The listing builds one solid part. Answer for the finished solid, in the listing's coordinates (mm). A direction names the side the tool comes from. Round coordinates to 2 decimals unless told otherwise and drop trailing zeros. Loops run counter-clockwise (first coordinate to the right, second up) from the corner with the lowest first, then second, coordinate; pieces in that order, holes last. Notation, with made-up numbers: (10.25, -23.5) -> (68.25, -23.5) arc R15 cw to (68.25, 0.5) -> close; hole circle Ø5 at (-6.5, -22). An arc over 180 degrees is marked (long way). Use a Markdown table: item, result. Add a question column.
Q1. Section C-C on y = -10 is taken. Give the vertices of the cut face in (x, z).
Q2. Given pin 1 Ø2 at (y, z) = (31.5, 4) entering from -X; pin 2 Ø3 at (y, z) = (14.5, -5.5) entering from -X; pin 3 Ø5 at (x, z) = (1.5, 4) entering from -Y, each flat-ended and moving along its own axis, determine where each tip first touches the part or whether it passes through.
Q3. Section D-D on z = -7 is taken. Give the vertices of the cut face in (x, y).
Q4. Section B-B on x = -2 is taken. Give the vertices of the cut face in (y, z).
Q5. Consider line 1 (Y direction, x = 0, z = -0.1); line 2 (Y direction, x = 4.5, z = -7); line 3 (Y direction, x = 2.25, z = 1). Determine where each line is inside the solid, lowest interval first.
Q6. Which of the six approach directions +Z, -Z, +X, -X, +Y, -Y give full straight-line access (tool end or side, diameter ignored) to faces 5 (the flat face through (0, -8, 0.75)), 6 (the flat face through (0, -12, 0)), 7 (the cylindrical face through (0.9, -0.99, -2.86))?
Q7. Section A-A on z = 0 is taken. Give the vertices of the cut face in (x, y).
Q8. For a pull along Y with two mould halves and no side action, classify faces 1 (the flat face through (0.1, 0, 3.4)), 2 (the flat face through (0, 39.5, 0)), 3 (the cylindrical face through (-0.108, -10.488, -0.31)), 4 (the cylindrical face through (-8.428, 28.092, 1.107)) as released by +Y, released by -Y, zero draft, split by the parting line, or undercut.
from build123d import *

# Parameters (mm, degrees)
SKETCH1_R               = 8
BOSS_EXTRUDE1_DEPTH     = 17
SKETCH2_R               = 8.5
BOSS_EXTRUDE2_DEPTH     = 22.5
SKETCH3_R               = 3
BOSS_EXTRUDE3_DEPTH     = 2
SKETCH4_R               = 1.4
BOSS_EXTRUDE4_DEPTH     = 10
CUT_EXTRUDE1_START      = -8.5
CUT_EXTRUDE1_DEPTH      = 8.5
CUT_EXTRUDE2_REACH      = 43.45
CUT_EXTRUDE2_END_RADIUS = 1.4
SKETCH6_R               = 0.5


with BuildPart() as part:
    # Sketch1 → Boss-Extrude1 (new body)
    with BuildSketch(Plane(origin=(0, 0, 0), x_dir=(1, 0, 0), z_dir=(0, 1, 0))):
        with Locations(Location((0, 0, 0), (0, 0, 270))):
            Circle(SKETCH1_R)
    extrude(amount=BOSS_EXTRUDE1_DEPTH)

    # Sketch2 → Boss-Extrude2 (add)
    with BuildSketch(Plane(origin=(0, 17, 0), x_dir=(1, 0, 0), z_dir=(0, 1, 0))):
        with Locations(Location((0, 0, 0), (0, 0, 90))):
            Circle(SKETCH2_R)
    extrude(amount=BOSS_EXTRUDE2_DEPTH)

    # Sketch3 → Boss-Extrude3 (add)
    with BuildSketch(Plane.XZ):
        with Locations(Location((0, 0, 0), (0, 0, 270))):
            Circle(SKETCH3_R)
    extrude(amount=BOSS_EXTRUDE3_DEPTH)

    # Sketch4 → Boss-Extrude4 (add)
    with BuildSketch(Plane.XZ.offset(2)):
        with Locations(Location((0, 0, 0), (0, 0, 270))):
            Circle(SKETCH4_R)
    extrude(amount=BOSS_EXTRUDE4_DEPTH)

    # Sketch5 → Cut-Extrude1 (cut)
    with BuildSketch(Plane.XZ.offset(12).offset(CUT_EXTRUDE1_START)):
        with BuildLine():
            Line((-1.182159042, 0.75), (1.182159042, 0.75))
            ThreePointArc((1.182159042, 0.75), (0, 1.4), (-1.182159042, 0.75))
        make_face()
    extrude(amount=CUT_EXTRUDE1_DEPTH, mode=Mode.SUBTRACT)

    # Cut-Extrude2: up to this cylinder (the profile starts inside it)
    cut_extrude2_end = Plane(origin=(0, -10, 0), z_dir=(0, 1, 0)) * Cylinder(CUT_EXTRUDE2_END_RADIUS, 90.7, mode=Mode.PRIVATE)
    # Sketch6 → Cut-Extrude2 (cut, up to the surface)
    with BuildSketch(Plane.XY.offset(0.75), mode=Mode.PRIVATE) as cut_extrude2_sk1:
        with Locations((0, -10)):
            Circle(SKETCH6_R)
    cut_extrude2_tool1 = extrude(cut_extrude2_sk1.sketch, amount=-CUT_EXTRUDE2_REACH, mode=Mode.PRIVATE) & cut_extrude2_end
    add(cut_extrude2_tool1.solids().sort_by_distance((0, -10, 0.75))[0], mode=Mode.SUBTRACT)


solid = part.part
Checked values:
| question | item | result |
|---|---|---|
| 1 | outline | (-1.18, 0.75) arc R1.4 ccw to (-0.5, -1.31) -> (-0.5, 0.75) -> close; (0.5, -1.31) arc R1.4 ccw to (1.18, 0.75) -> (0.5, 0.75) -> close |
| 2 | pin 1 | stops at x = -7.95 |
| 2 | pin 2 | stops at x = -6.93 |
| 2 | pin 3 | stops at y = -2 |
| 3 | outline | (-4.82, 17) -> (-3.87, 17) -> (-3.87, 0) -> (3.87, 0) -> (3.87, 17) -> (4.82, 17) -> (4.82, 39.5) -> (-4.82, 39.5) -> close |
| 4 | outline | (-2, -2.24) -> (0, -2.24) -> (0, -7.75) -> (17, -7.75) -> (17, -8.26) -> (39.5, -8.26) -> (39.5, 8.26) -> (17, 8.26) -> (17, 7.75) -> (0, 7.75) -> (0, 2.24) -> (-2, 2.24) -> close |
| 5 | line 1 | y = -12 to -10.5, -9.5 to 39.5 |
| 5 | line 2 | y = 17 to 39.5 |
| 5 | line 3 | y = -2 to 39.5 |
| 6 | face 5 | +Z, +X, -X, -Y |
| 6 | face 6 | +Z, -Z, +X, -X, -Y |
| 6 | face 7 | -Y |
| 7 | outline | (-8.5, 17) -> (-8, 17) -> (-8, 0) -> (-3, 0) -> (-3, -2) -> (-1.4, -2) -> (-1.4, -12) -> (1.4, -12) -> (1.4, -2) -> (3, -2) -> (3, 0) -> (8, 0) -> (8, 17) -> (8.5, 17) -> (8.5, 39.5) -> (-8.5, 39.5) -> close; hole circle Ø1 at (0, -10) |
| 8 | face 1 | released by -Y |
| 8 | face 2 | released by +Y |
| 8 | face 3 | undercut |
| 8 | face 4 | zero draft |
